Work out the finished part from the listing and answer in its coordinate system (mm). A direction names the side the tool comes from. Coordinates: 2 decimals unless noted, no trailing zeros. Write each loop counter-clockwise with the first axis right and the second up, starting at its lowest first coordinate (ties: lowest second). Pieces come first, ordered by that corner, then holes. Notation, with made-up numbers: (47.25, 62) -> (97.25, 62) arc R10 ccw to (97.25, 79) -> close; hole circle Ø11 at (-11.5, 73). An arc over 180 degrees is marked (long way). Write each question's results on one line, items separated by ' | '. Start each with the question number.
Solid Edge part; units mm, degrees
sketch "Sketch1" plane through (0, 0, 0) normal (0, -1, 0) x (1, 0, 0)
  line L0 (0, -25) -> (1.5, -25)
  line L1 (1.5, -25) -> (1.5, -7)
  arc A0 (1.5, -6.99) -> (1.5, -7) centre (1.5038, -6.995) ccw
  line L2 (1.5, -6.99) -> (1.5, 0)
  line L3 (1.5, 0) -> (2.85, 0)
  line L4 (2.85, 0) -> (2.85, 0.165)
  arc A1 (1.27, 1.65) -> (2.85, 0.165) centre (-0.3628, -1.6703) cw
  line L5 (0, 1.65) -> (1.27, 1.65)
  dimension "D1" = 1.5
revolve "RevolvedProtrusion1" add sketch "Sketch1" angle 360 about axis through (0, 0, 5) along (0, 0, -1)
sketch "Sketch2" plane through (0, 0, 0) normal (0, -1, 0) x (1, 0, 0)
  line L0 (0, -0.0566) -> (1.1545, 0.61)
  line L1 (1.1545, 0.61) -> (1.1545, 1.65)
  line L2 (1.1545, 1.65) -> (0, 1.65)
revolve "RevolvedCutout1" cut sketch "Sketch2" angle 360 about axis through (0, 0, 5.3) along (0, 0, -1)
sketch "Sketch3" plane through (0, 0, 0) normal (0, 0, -1) x (0, 1, 0)
  arc A0 (-1, 0.577) -> (-1, -0.577) centre (0, 0) ccw
  line L0 (-1, 0.577) -> (-1, -0.577)
extrude "Protrusion1" add sketch "Sketch3" against normal blind 1.65
pattern_circular "Pattern1" count 6 over 360 about axis through (0, 0, 0) along (0, 0, -1) of "Protrusion1"
fillet "Round_1" radius 0.185 1 edges at (-1.27, 0, 1.65)
sketch "Sketch4" plane through (0, 0, 0) normal (0, -1, 0) x (1, 0, 0)
  line L0 (0, 0.9501) -> (1.2122, 1.65)
  line L1 (1.2122, 1.65) -> (0, 1.65)
revolve "RevolvedCutout2" cut sketch "Sketch4" angle 360 about axis through (0, 0, 5.3) along (0, 0, -1)
sketch "Sketch5" plane through (0, 0, 0) normal (0, -1, 0) x (1, 0, 0)
  line L0 (-1.5, 0) -> (-1.5, -0.1)
  line L1 (-1.6, 0) -> (-1.5, 0)
  arc A0 (-1.6, 0) -> (-1.5, -0.1) centre (-1.6, -0.1) cw
revolve "RevolvedProtrusion2" add sketch "Sketch5" angle 360 about axis through (0, 0, -0.5) along (0, 0, 1)
cosmetic_thread "Thread1"
chamfer "Chamfer1" distance 0.3065 angle 45 1 edges at (-1.5, 0, -25)
properties material "Stahl"
1. For faces 1 (the face through (-1.5, 0.07, -15.72)), 2 (the face through (0, 0, -25)), 3 (the face through (0, -1, 1)), determine the directions among +Z, -Z, +X, -X, +Y, -Y from which every point of the face is accessible in a straight line to the end or side of a thin tool.
2. Find the intervals of material crossed by L1, parallel to Y at x = 0.9, z = -10; L2, parallel to Z at x = -0.45, y = -1.1; L3, parallel to Z at x = -1.1, y = -2.3, in increasing order.
3. Find section A-A on z = -7.75. Give the vertices of the cut face in (x, y).
4. Given pin 1 Ø0.9 at (x, z) = (0.5, 1) entering from -Y; pin 2 Ø2 at (y, z) = (1.5, -16.5) entering from -X; pin 3 Ø1 at (x, z) = (0, -6.5) entering from -Y, each flat-ended and moving along its own axis, determine where each tip first touches the part or whether it passes through.
Ans:
1) face 1: -Z | face 2: -Z, +X, -X, +Y, -Y | face 3: +Z
2) L1: y = -1.2 to 1.2 | L2: z = -25 to 1.64 | L3: z = 0 to 0.61
3) outline: circle Ø3 at (0, 0)
4) pin 1: stops at y = -2.56 | pin 2: stops at x = -1.41 | pin 3: stops at y = -1.5
